Design review of the part built by this model. Coordinates are the model's own, in mm. Give positions to 0.01 mm unless a question says otherwise; leave off trailing zeros. Order: outer loops, then holes, each group sorted by start corner. A loop starts at its lowest first (then second) coordinate and runs counter-clockwise, first axis right, second up. Notation, with made-up numbers: (1.25, 40) - (19.25, 40) arc R35 cw to (19.25, 76) - close; hole circle Ø2 at (-23, 28.5). An arc over 180 degrees is marked (long way). Write each question's results on one line, items separated by ' | '. Start each with the question number.
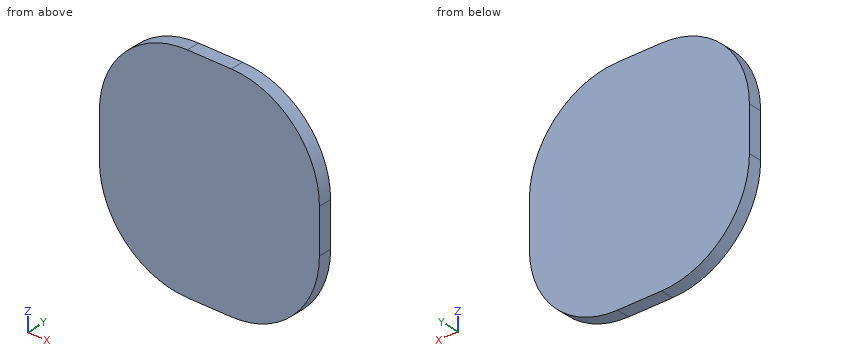
Autodesk Inventor part; units mm, degrees
ref_plane "YZ Plane" through (0, 0, 0) normal (1, 0, 0) x (0, 1, 0)
ref_plane "XZ Plane" through (0, 0, 0) normal (0, 1, 0) x (-1, 0, 0)
ref_plane "XY Plane" through (0, 0, 0) normal (0, 0, 1) x (1, 0, 0)
sketch "Sketch1" plane through (0, 0, 0) normal (0, 1, 0) x (-1, 0, 0)
  line L0 (15, -15) -> (-35, -15)
  line L1 (-35, -15) -> (-35, 35)
  line L2 (-35, 35) -> (15, 35)
  line L3 (15, 35) -> (15, -15)
  line L4 (15, -15) -> (-35, 35) construction
  line L5 (-35, -15) -> (15, 35) construction
  point P0 (-10, 10)
  dimension "d2" = 50
  dimension "d3" = 50
extrude "Extrusion1" add sketch "Sketch1" along normal blind 3
fillet "Fillet1" radius 20 4 edges at (35, 1.5, 35) (-15, 1.5, 35) (-15, 1.5, -15) (35, 1.5, -15)
equation "\"d2\" = d3"
properties part number "power-bank-bump"
Q1. Insertion check: pin 1 Ø1.5 at (x, y) = (26.5, 2) entering from +Z. The pin has a flat end and moves straight along its axis. Give the tip position at first contact, or say it passes through.
Q2. Add section B-B (x = 31). Give the boundary of the cut face in (y, z).
Q3. Add section C-C (z = -1). Give the boundary of the cut face in (x, y), plus the area to 3 significant figures.
Q4. Add section A-A (y = 2.2). Give the boundary of the cut face in (x, z).
Q5. For line 1 (X direction, y = 1.75, z = 15.5); line 2 (Z direction, x = -1, y = 0.3); line 3 (X direction, y = 1.7, z = 16.5), list the stretches that pass through material, from the lowest coordinate up. Write a range as [from, to].
Verdict:
1) pin 1: stops at z = 31.87
2) outline: (0, -7) - (3, -7) - (3, 27) - (0, 27) - close
3) outline: (-14.08, 0) - (34.08, 0) - (34.08, 3) - (-14.08, 3) - close | area: 144 mm2
4) outline: (-15, 5) arc R20 ccw to (5, -15) - (15, -15) arc R20 ccw to (35, 5) - (35, 15) arc R20 ccw to (15, 35) - (5, 35) arc R20 ccw to (-15, 15) - close
5) line 1: x = [-14.99, 34.99] | line 2: z = [-14.08, 34.08] | line 3: x = [-14.94, 34.94]
